The listing builds one solid part. Answer for the finished solid, in the listing's coordinates (mm). A direction names the side the tool comes from. Give positions to 0.01 mm unless a question says otherwise; leave off trailing zeros. Order: outer loops, then holes, each group sorted by start corner. A loop starts at its lowest first (then second) coordinate and runs counter-clockwise, first axis right, second up. Notation, with made-up numbers: (23.5, 27) - (37.5, 27) arc R23 ccw to (37.5, 54) - close; hole circle Ø2 at (1.5, 15.25). An arc over 180 degrees is marked (long way). Answer as a JSON object with one key per item and string values. Group by question number.
Q1. For faces 1 (the face through (13.887, 10.648, -234.227)), 2 (the face through (-2, 18, 2.5)), 3 (the face through (0, 15, -187)), determine the directions among +Z, -Z, +X, -X, +Y, -Y from which every point of the face is accessible in a straight line to the end or side of a thin tool.
Q2. The mould has two halves that part along X. Classify faces 4 (the face through (-4.336, -19.524, -79.235)), 5 (the face through (18, 6, -160)), 6 (the face through (0, 18, -165)): released by +X, released by -X, zero draft, split by the parting line, or undercut.
Q3. A cutting plane is placed at B-B, the plane z = -233. Give the vertices of the cut face in (x, y).
Q4. A cutting plane is placed at A-A, the plane z = -33.5. Give the vertices of the cut face in (x, y), and give its area (3 significant figures).
Q5. Given pin 1 (1 mm diameter, centred on x = 12.5, y = 19.5, fed in from +Z); pin 2 (4.5 mm diameter, centred on y = 16.5, z = -180.5, fed in from +X); pin 3 (1.2 mm diameter, centred on y = 16.5, z = -192.5, fed in from -X), each flat-ended and moving along its own axis, determine where each tip first touches the part or whether it passes through.
Q6. A cutting plane is placed at C-C, the plane z = -194.5. Give the vertices of the cut face in (x, y), and give its area (3 significant figures).
Q7. Consider line 1 (Z direction, x = -1, y = 15.5); line 2 (Z direction, x = -6.5, y = -19); line 3 (Y direction, x = 0.5, z = -27). Determine where each line is inside the solid, lowest interval first.
Autodesk Inventor part; units mm, degrees
ref_plane "Plano de trabalho2" through (0, 20, 0) normal (0, 1, 0) x (-1, 0, 0)
ref_plane "YZ Plane" through (0, 0, 0) normal (1, 0, 0) x (0, 1, 0)
ref_plane "XY Plane" through (0, 0, 0) normal (0, 0, 1) x (1, 0, 0)
sketch "Esboço1" plane through (0, 0, 0) normal (0, 0, 1) x (-1, 0, 0)
  circle A0 centre (0, 0) radius 25
  dimension "d0" = 50
extrude "Extrusão1" add sketch "Esboço1" along normal mid plane 5
sketch "Esboço2" plane through (0, 0, 0) normal (0, 0, -1) x (1, 0, 0)
  circle A0 centre (0, 0) radius 20
  dimension "d3" = 40
extrude "Extrusão2" add sketch "Esboço2" along normal blind 215
sketch "Esboço3" plane through (0, 0, 0) normal (0, 0, 1) x (1, 0, 0)
  circle A0 centre (0, 0) radius 17.5
  dimension "d6" = 35
extrude "Extrusão3" add sketch "Esboço3" along normal blind 29
chamfer "Chanfro2" distance 1 angle 45 3 edges at (25, 0, -2.5) (25, 0, 2.5) (-17.5, 0, 29)
ref_plane "Plano de trabalho2" through (0, 20, 0) normal (0, 1, 0) x (-1, 0, 0)
sketch "Esboço7" plane through (0, 20, 0) normal (0, 1, 0) x (-1, 0, 0)
  line L0 (0, -63) -> (0, -43) construction
  line L1 (6, -63) -> (6, -43)
  line L2 (-6, -43) -> (-6, -63)
  arc A0 (-6, -63) -> (6, -63) centre (0, -63) ccw
  arc A1 (6, -43) -> (-6, -43) centre (0, -43) ccw
  line L3 (24, -2.5) -> (-24, -2.5)
  point P0 (0, 0)
  point P1 (0, -53)
  dimension "d25" = 12
  dimension "d26" = 20
  dimension "d27" = 40.5
extrude "Extrusão6" cut sketch "Esboço7" against normal blind 5
sketch "Esboço8" plane through (0, 0, -215) normal (0, 0, -1) x (-1, 0, 0)
  circle A0 centre (0, 0) radius 20
  circle A1 centre (0, 0) radius 17.5
  dimension "d30" = 35
extrude "Extrusão7" add sketch "Esboço8" along normal blind 3 contours A1
sketch "Esboço9" plane through (0, 0, -218) normal (0, 0, -1) x (-1, 0, 0)
  circle A0 centre (0, 0) radius 17.5
  circle A1 centre (0, 0) radius 19.5
  dimension "d33" = 39
extrude "Extrusão8" add sketch "Esboço9" along normal blind 38 contours A0
chamfer "Chanfro3" distance 2 angle 45 1 edges at (17.5, 0, -256)
thread "Rosca1"
sketch "Esboço10" plane through (0, 0, 0) normal (1, 0, 0) x (0, 1, 0)
  line L0 (20, -2.5) -> (20, -215)
  line L1 (20, -160) -> (18.75, -160)
  line L2 (18.75, -160) -> (18.75, -158.15)
  line L3 (18.75, -158.15) -> (20, -158.15)
  line L4 (20, -158.15) -> (20, -160)
  line L5 (0, 0) -> (0, -179.7731)
  dimension "d41" = 1.85
  dimension "d42" = 160
  dimension "d43" = 37.5
revolve "Revolução1" cut sketch "Esboço10" angle 360 about axis through (0, 0, 0) along (0, 0, -1)
sketch "Esboço11" plane through (0, 20, 0) normal (0, 1, 0) x (-1, 0, 0)
  line L0 (0, -204) -> (0, -171) construction
  line L1 (6, -204) -> (6, -171)
  line L2 (-6, -171) -> (-6, -204)
  arc A0 (-6, -204) -> (6, -204) centre (0, -204) ccw
  arc A1 (6, -171) -> (-6, -171) centre (0, -171) ccw
  point P0 (0, 0)
  point P1 (0, -187.5)
  dimension "d45" = 171
  dimension "d46" = 33
  dimension "d47" = 6
extrude "Extrusão9" cut sketch "Esboço11" against normal blind 5
properties material "Liga de aço"
Reply:
{
 "1": {"face 1": "-Z", "face 2": "+Z", "face 3": "+Y"},
 "2": {"face 4": "split by the parting line", "face 5": "zero draft", "face 6": "undercut"},
 "3": {"outline": "circle Ø35 at (0, 0)"},
 "4": {"outline": "circle Ø40 at (0, 0)", "area": "1,260 mm^2"},
 "5": {"pin 1": "stops at z = 2.5", "pin 2": "stops at x = 14.03", "pin 3": "stops at x = -12.13"},
 "6": {"outline": "(-6, 15) - (-6, 19.08) arc R20 ccw (long way) to (6, 19.08) - (6, 15) - close", "area": "1,200 mm^2"},
 "7": {"line 1": "z = -255.97 to -209.92, -165.08 to -68.92, -37.08 to 29", "line 2": "z = -2.5 to 2.5", "line 3": "y = -19.99 to 19.99"}
}
